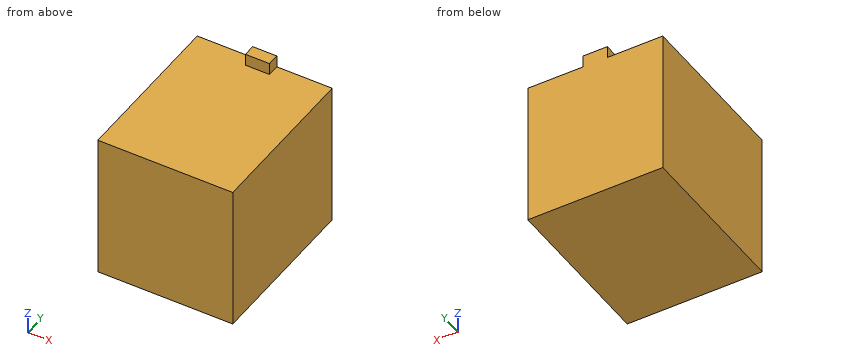
```python
from build123d import *

# Parameters (mm, degrees)
SKETCH_1_W      = 56.1
SKETCH_1_H      = 60.6
EXTRUDE_1_DEPTH = 68
SKETCH_2_W      = 5
SKETCH_2_H      = 5
EXTRUDE_2_DEPTH = 5


with BuildPart() as part:
    # 草图1 → 凸台-拉伸1 (new body)
    with BuildSketch(Plane(origin=(0, 0, 0), x_dir=(1, 0, 0), z_dir=(0, 1, 0))):
        Rectangle(SKETCH_1_W, SKETCH_1_H)
    extrude(amount=EXTRUDE_1_DEPTH)

    # 草图2 → 凸台-拉伸2 (add)
    with BuildSketch(Plane.XY.offset(30.3)):
        with Locations((-2.5, 65.5)):
            Rectangle(SKETCH_2_W, SKETCH_2_H)
        with Locations((2.5, 65.5)):
            Rectangle(SKETCH_2_W, SKETCH_2_H)
    extrude(amount=EXTRUDE_2_DEPTH)


solid = part.part
```
Verification items for the finished model (mm, model axes). Coordinates: 2 decimals unless noted, no trailing zeros. Order: outer loops, then holes, each group sorted by start corner. A loop starts at its lowest first (then second) coordinate and runs counter-clockwise, first axis right, second up. Notation, with made-up numbers: (31.5, 37.25) -> (51.5, 37.25) arc R28 ccw to (51.5, 64.25) -> close; hole circle Ø8 at (-6, 55). An arc over 180 degrees is marked (long way). Put each result on its own line as item: value. Start each with the question number.
1) Cross-section at C-C (x = -1). Enter the section's corners in (y, z), plus the area to 3 significant figures.
2) Cross-section at B-B (y = 31). Enter the section's corners in (x, z), plus the area to 3 significant figures.
3) Go/stop test with flat-tipped pins: pin 1 (5 mm diameter, centred on x = 3.5, z = 20.5, fed in from -Y); pin 2 (3 mm diameter, centred on x = 2.5, y = 22, fed in from +Z); pin 3 (2.5 mm diameter, centred on y = 65, z = 33.5, fed in from +X); pin 4 (1.5 mm diameter, centred on y = 65, z = 32.5, fed in from -X). Record where each tip stops, or that it passes through.
4) Material ranges on L1, parallel to Z at x = -20.5, y = 19.5, recorded low to high.
5) Cross-section at A-A (x = -13). Enter the section's corners in (y, z), plus the area to 3 significant figures.
Geometry check:
1. outline: (0, -30.3) -> (68, -30.3) -> (68, 35.3) -> (63, 35.3) -> (63, 30.3) -> (0, 30.3) -> close
1. area: 4,150 mm^2
2. outline: (-28.05, -30.3) -> (28.05, -30.3) -> (28.05, 30.3) -> (-28.05, 30.3) -> close
2. area: 3,400 mm^2
3. pin 1: stops at y = 0
3. pin 2: stops at z = 30.3
3. pin 3: stops at x = 5
3. pin 4: stops at x = -5
4. L1: z = -30.3 to 30.3
5. outline: (0, -30.3) -> (68, -30.3) -> (68, 30.3) -> (0, 30.3) -> close
5. area: 4,120 mm^2
